```python
from build123d import *

# Parameters (mm, degrees)
ESQUISSE1_R             = 6
ESQUISSE1_R_2           = 2.25
BOSS_EXTRU_1_DEPTH      = 10
ESQUISSE2_W             = 1
ESQUISSE2_H             = 2
ENL_V_MAT_EXTRU_1_DEPTH = 20
ESQUISSE3_W             = 2.690646438
ESQUISSE3_H             = 2.455091602
ENL_V_MAT_EXTRU_2_DEPTH = 3


with BuildPart() as part:
    # Esquisse1 → Boss.-Extru.1 (new body)
    with BuildSketch(Plane(origin=(0, 0, 0), x_dir=(1, 0, 0), z_dir=(0, 1, 0))):
        with Locations(Location((0, 0, 0), (0, 0, 270))):
            Circle(ESQUISSE1_R)
        with Locations(Location((0, 0, 0), (0, 0, 270))):
            Circle(ESQUISSE1_R_2, mode=Mode.SUBTRACT)
    extrude(amount=BOSS_EXTRU_1_DEPTH)

    # Esquisse2 → Enlèv. mat.-Extru.1 (cut)
    with BuildSketch(Plane(origin=(0, 10, 0), x_dir=(1, 0, 0), z_dir=(0, 1, 0))):
        with Locations((0, -6)):
            Rectangle(ESQUISSE2_W, ESQUISSE2_H)
    extrude(amount=-ENL_V_MAT_EXTRU_1_DEPTH, mode=Mode.SUBTRACT)

    # Esquisse3 → Enlèv. mat.-Extru.2 (cut)
    with BuildSketch(Plane(origin=(0, 10, 0), x_dir=(1, 0, 0), z_dir=(0, 1, 0))):
        with Locations((0, -5)):
            Rectangle(ESQUISSE3_W, ESQUISSE3_H)
    extrude(amount=-ENL_V_MAT_EXTRU_2_DEPTH, mode=Mode.SUBTRACT)


solid = part.part
```
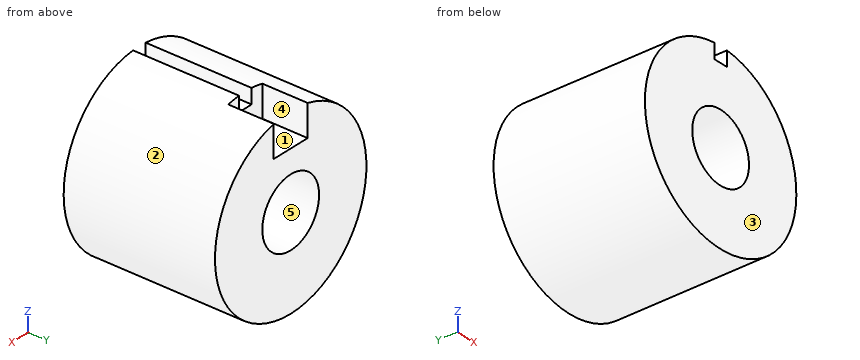
Input: part model. Units: mm. Frame: model coordinates. Face numbers are marked on the shaded views. A direction names the side the tool comes from. Round coordinates to 2 decimals unless told otherwise and drop trailing zeros. Loops run counter-clockwise (first coordinate to the right, second up) from the corner with the lowest first, then second, coordinate; pieces in that order, holes last. Notation, with made-up numbers: (-5, 73) -> (42, 73) arc R4 cw to (42, 79) -> close; hole circle Ø1 at (-29, 50). An arc over 180 degrees is marked (long way). One line per item, written item: value.
(1) Material intervals for line 1 (X direction, y = 6.25, z = 0); line 2 (X direction, y = 3.25, z = 0.75); line 3 (X direction, y = 3, z = -4), sorted ascending. Write a range as [from, to].
Geometry check:
line 1: [-6, -2.25], [2.25, 6]
line 2: [-5.95, -2.12], [2.12, 5.95]
line 3: [-4.47, 4.47]
(2) Mould query, pull axis X, two halves, no side actions, for the marked faces 1, 2 and 3. Classes: pulls with the +X half, pulls with the -X half, needs draft (parallel to the pull), parting line crosses it, or undercut.
Geometry check:
face 1: undercut
face 2: parting line crosses it
face 3: needs draft
(3) Section A-A (x = 0). Return the cut outline in (y, z), plus the area to 3 significant figures.
Geometry check:
outline: (0, -6) -> (10, -6) -> (10, -2.25) -> (0, -2.25) -> close; (0, 2.25) -> (10, 2.25) -> (10, 3.77) -> (7, 3.77) -> (7, 5) -> (0, 5) -> close
area: 61.3 mm2
(4) Section C-C (y = 4.5). Return the cut outline in (x, z).
Geometry check:
outline: (-0.5, 5) -> (-0.5, 5.98) arc R6 ccw (long way) to (0.5, 5.98) -> (0.5, 5) -> close; hole circle Ø4.5 at (0, 0)
(5) Pin query (flat end, axial travel): pin 1 (1.1 mm diameter, centred on y = 4, z = 5.5, fed in from +X); pin 2 (0.5 mm diameter, centred on y = 3, z = 5.5, fed in from -X); pin 3 (2.5 mm diameter, centred on y = 9, z = 5, fed in from +X). Return the tip coordinate at first contact, or that it passes through.
Geometry check:
pin 1: x = 3.39
pin 2: x = -2.9
pin 3: x = 4.68
(6) Section D-D (y = 8.5). Return the cut outline in (x, z).
Geometry check:
outline: (-1.35, 3.77) -> (-1.35, 5.85) arc R6 ccw (long way) to (1.35, 5.85) -> (1.35, 3.77) -> close; hole circle Ø4.5 at (0, 0)
(7) Set-up query: the marked faces 4 and 5. Return all of +Z, -Z, +X, -X, +Y, -Y with unobstructed straight access to the full face (end or side cutting, diameter ignored); none if empty.
Geometry check:
face 4: +Z, +Y
face 5: +Y, -Y
(8) Section B-B (z = 0). Return the cut outline in (x, y), plus the area to 3 significant figures.
Geometry check:
outline: (-6, 0) -> (-2.25, 0) -> (-2.25, 10) -> (-6, 10) -> close; (2.25, 0) -> (6, 0) -> (6, 10) -> (2.25, 10) -> close
area: 75.0 mm2
